```python
from build123d import *

# Parameters (mm, degrees)
F1_DEPTH = 60
F3_DEPTH = 106.9
F5_DEPTH = 25


with BuildPart() as f1:
    # F0 (on Top) → F1 (new body)
    with BuildSketch(Plane.XY):
        with BuildLine():
            Line((0, 5), (0, 0))
            Line((0, 0), (35, 0))
            ThreePointArc((35, 0), (42.071068, 2.928932), (45, 10))
            Line((45, 10), (45, 40))
            ThreePointArc((45, 40), (46.464466, 43.535534), (50, 45))
            Line((50, 45), (110, 45))
            Line((110, 45), (110, 50))
            Line((110, 50), (50, 50))
            ThreePointArc((50, 50), (42.928932, 47.071068), (40, 40))
            Line((40, 40), (40, 10))
            ThreePointArc((40, 10), (38.535534, 6.464466), (35, 5))
            Line((35, 5), (0, 5))
        make_face()
    extrude(amount=F1_DEPTH)

    # F2 (on face) → F3 (cut)
    with BuildSketch(Plane.XZ):
        with BuildLine():
            ThreePointArc((24.5, 10), (23.181981, 13.181981), (20, 14.5))
            ThreePointArc((20, 14.5), (16.818019, 6.818019), (24.5, 10))
        make_face()
        with BuildLine():
            ThreePointArc((24.5, 50), (23.181981, 53.181981), (20, 54.5))
            Line((20, 54.5), (20, 50))
            Line((20, 50), (20, 45.5))
            ThreePointArc((20, 45.5), (23.181981, 46.818019), (24.5, 50))
        make_face()
        with BuildLine():
            Line((20, 50), (20, 54.5))
            ThreePointArc((20, 54.5), (15.5, 50), (20, 45.5))
            Line((20, 45.5), (20, 50))
        make_face()
        with BuildLine():
            ThreePointArc((100.5, 30), (95, 35.5), (89.5, 30))
            ThreePointArc((89.5, 30), (95, 24.5), (100.5, 30))
        make_face()
        with BuildLine():
            ThreePointArc((70.5, 30), (68.889087, 33.889087), (65, 35.5))
            Line((65, 35.5), (65, 30))
            Line((65, 30), (70.5, 30))
        make_face()
        with BuildLine():
            Line((65, 30), (65, 35.5))
            ThreePointArc((65, 35.5), (61.110913, 26.110913), (70.5, 30))
            Line((70.5, 30), (65, 30))
        make_face()
    extrude(amount=-F3_DEPTH, mode=Mode.SUBTRACT)

    # F4 (on face) → F5 (cut)
    with BuildSketch(Plane(origin=(40, 0, 0), x_dir=(0, -1, 0), z_dir=(-1, 0, 0))):
        with BuildLine():
            ThreePointArc((-35, 30), (-30, 25), (-25, 30))
            ThreePointArc((-25, 30), (-30, 35), (-35, 30))
        make_face()
    extrude(amount=-F5_DEPTH, mode=Mode.SUBTRACT)


solid = f1.part
```
Could you check a few things on this model? Use its own coordinates, in mm. A direction names the side the tool comes from. Coordinates: 2 decimals unless noted, no trailing zeros. Write each loop counter-clockwise with the first axis right and the second up, starting at its lowest first coordinate (ties: lowest second). Pieces come first, ordered by that corner, then holes. Notation, with made-up numbers: (63.25, 37.25) -> (102.25, 37.25) arc R23 cw to (102.25, 74.25) -> close; hole circle Ø6 at (40.5, -12). An arc over 180 degrees is marked (long way). Write item = value, one per line. Start each with the question number.
(1) I need wall thicknesses on line 1 (Z direction, x = 20, y = 2.2); line 2 (X direction, y = 48.2, z = 30); line 3 (Z direction, x = 65, y = 48.7). Which ranges of each line are inside material? Lowest first, please. Write a range as [from, to].
(2) I want a section at D-D (z = 27). Please give me the cut outline in (x, y), plus the area to 3 significant figures.
(3) Which directions (+Z, -Z, +X, -X, +Y, -Y) give clear straight access to the entire face, cutting with the end or side of a thin tool? Please do faces 1 (the face through (45, 24.8, 29.6)), 2 (the face through (40, 22, 30)), 3 (the face through (110, 47, 30)).
(4) I want a section at B-B (z = 39.5). Please give me the cut outline in (x, y), plus the area to 3 significant figures.
(5) We'd pull the mould along X, two halves only. Please class faces 4 (the face through (100.495, 47.465, 29.758)), 5 (the face through (42, 34, 27)), 6 (the face through (43.01, 47.15, 29.58)): released by +X, released by -X, zero draft, split by the parting line, or undercut.
(6) I want a section at A-A (y = 30). Please give me the cut outline in (x, z).
(7) Will these pins go through, and if not, where does the flat tip stop? pin 1 (12 mm diameter, centred on y = 10.5, z = 29, fed in from +X); pin 2 (7 mm diameter, centred on x = 20, z = 10, fed in from -Y); pin 3 (13 mm diameter, centred on y = 30, z = 30, fed in from -X); pin 4 (17.5 mm diameter, centred on x = 95, z = 30, fed in from -Y).
(8) I want a section at C-C (x = 95). Please give me the cut outline in (y, z), plus the area to 3 significant figures.
Result set:
q1.line_1 = [0, 5.5], [14.5, 45.5], [54.5, 60]
q1.line_2 = [44.28, 59.5], [70.5, 89.5], [100.5, 110]
q1.line_3 = [0, 24.5], [35.5, 60]
q2.outline = (0, 0) -> (35, 0) arc R10 ccw to (45, 10) -> (45, 26) -> (40, 26) -> (40, 10) arc R5 cw to (35, 5) -> (0, 5) -> close; (40, 34) -> (45, 34) -> (45, 40) arc R5 cw to (50, 45) -> (60.39, 45) -> (60.39, 50) -> (50, 50) arc R10 ccw to (40, 40) -> close; (69.61, 45) -> (90.39, 45) -> (90.39, 50) -> (69.61, 50) -> close; (99.61, 45) -> (110, 45) -> (110, 50) -> (99.61, 50) -> close
q2.area = 611 mm2
q3.face_1 = +Z, -Z, +X, -Y
q3.face_2 = +Z, -Z, -X, +Y
q3.face_3 = +Z, -Z, +X, +Y, -Y
q4.outline = (0, 0) -> (35, 0) arc R10 ccw to (45, 10) -> (45, 40) arc R5 cw to (50, 45) -> (110, 45) -> (110, 50) -> (50, 50) arc R10 ccw to (40, 40) -> (40, 10) arc R5 cw to (35, 5) -> (0, 5) -> close
q4.area = 743 mm2
q5.face_4 = undercut
q5.face_5 = zero draft
q5.face_6 = released by -X
q6.outline = (40, 0) -> (45, 0) -> (45, 25) -> (40, 25) -> close; (40, 35) -> (45, 35) -> (45, 60) -> (40, 60) -> close
q7.pin_1 = 45
q7.pin_2 = through
q7.pin_3 = 40
q7.pin_4 = 45
q8.outline = (45, 0) -> (50, 0) -> (50, 24.5) -> (45, 24.5) -> close; (45, 35.5) -> (50, 35.5) -> (50, 60) -> (45, 60) -> close
q8.area = 245 mm2
